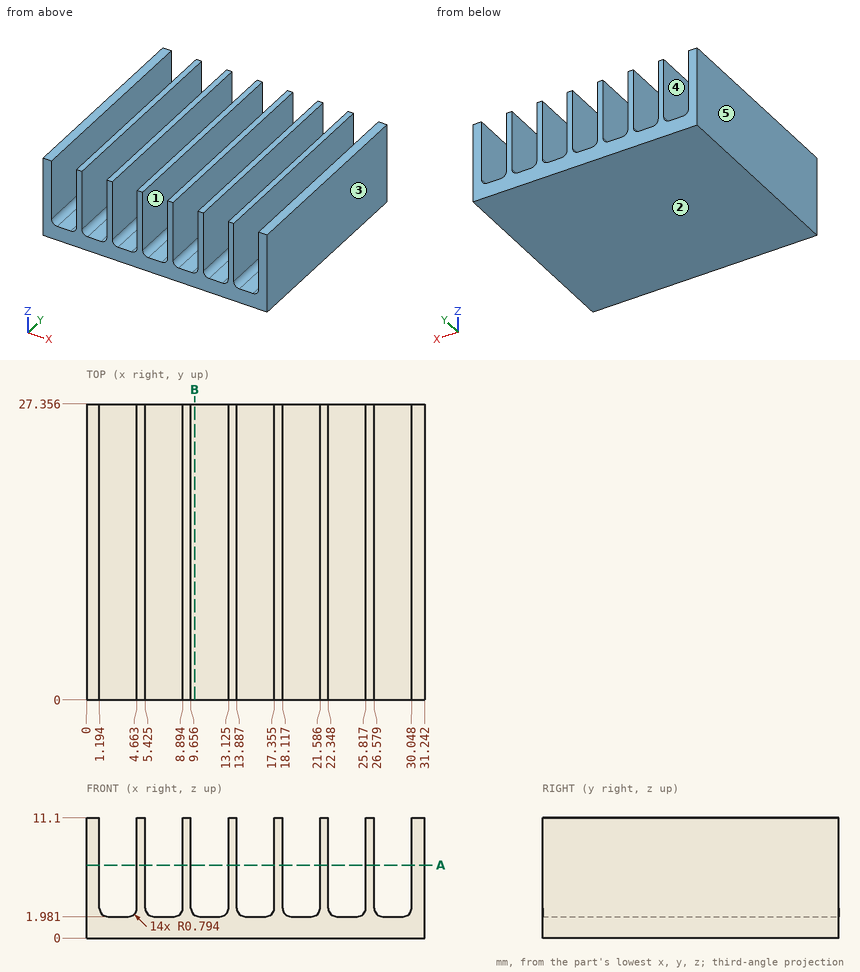
Answer from the drawing. Dimensions are ordinates in mm from the lowest x, y and z of the part. A direction names the side the tool comes from. Give positions to 0.01 mm unless a question says otherwise; leave off trailing zeros. Write each loop counter-clockwise with the first axis right and the second up, starting at its lowest first coordinate (ties: lowest second). Pieces come first, ordered by that corner, then holes. Notation, with made-up numbers: (-3.75, -34.75) -> (52.25, -34.75) arc R22 cw to (52.25, -6.75) -> close; hole circle Ø7 at (-4, 73.25). An arc over 180 degrees is marked (long way). Use a Markdown table: item, result.
(1) Determine the mould class of the marked faces 1, 2 and 3 for opening direction X: released by +X, released by -X, zero draft, split by the parting line, or undercut.
Return value:
| item | result |
|---|---|
| face 1 | undercut |
| face 2 | zero draft |
| face 3 | released by +X |
(2) Section A-A, the plane z = 6.75 is taken. Give the number of separate pieces and of enclosed holes in the cut face.
Return value:
| item | result |
|---|---|
| separate pieces | 8 |
| enclosed holes | 0 |
(3) Find the intervals of material crossed by probe 1 along Z at (x, y) = (24, 12); probe 2 along Z at (x, y) = (27, 3.25) (1 decimal), in increasing order. Write a range as from..to.
Return value:
| item | result |
|---|---|
| probe 1 | 0..1.98 |
| probe 2 | 0..2.1 |
(4) Section B-B, the plane x = 10 is taken. Determine the outline of the cut face in (y, z) (1 decimal).
Return value:
| item | result |
|---|---|
| outline | (0, 0) -> (27.4, 0) -> (27.4, 2.1) -> (0, 2.1) -> close |
(5) For the marked faces 4 and 5, determine the directions among +Z, -Z, +X, -X, +Y, -Y from which every point of the face is accessible in a straight line to the end or side of a thin tool.
Return value:
| item | result |
|---|---|
| face 4 | +Z, +Y, -Y |
| face 5 | +Z, -Z, -X, +Y, -Y |
(6) A flat-ended cylindrical pin translates along its axis: P1, Ø1.5, axis at x = 11.5, y = 8.5, coming from the +Z side. Find the tip coordinate at first contact, or state that the pin passes through.
Return value:
| item | result |
|---|---|
| P1 | z = 1.98 |
